```python
from build123d import *

# Parameters (mm, degrees)
EXTRUDE_1_DEPTH = 10
EXTRUDE_2_DEPTH = 2.5
EXTRUDE_3_DEPTH = 2.5


with BuildPart() as part:
    # 草图1 → 凸台-拉伸1 (new body)
    with BuildSketch(Plane.XY):
        Polygon((-6, -2.715432056), (-6, -10.574613101), (-11, -10.574613101), (-11, 19.425386899), (-5, 19.425386899), (5, 19.425386899), (11, 19.425386899), (11, -10.574613101), (6, -10.574613101), (6, -2.715432056), (7, -2.715432056), (7, 14.925386899), (-7, 14.925386899), (-7, -2.715432056), align=None)
    extrude(amount=EXTRUDE_1_DEPTH)

    # 草图2 → 凸台-拉伸2 (add)
    with BuildSketch(Plane(origin=(0, 0, 0), x_dir=(0, 0, -1), z_dir=(1, 0, 0))):
        Polygon((-10, 19.425386899), (-10, 31.425386899), (-14.821209098, 31.425386899), (-14.821209098, 33.063700588), (4.821209098, 33.063700588), (4.821209098, 31.425386899), (0, 31.425386899), (0, 19.425386899), align=None)
    extrude(amount=EXTRUDE_2_DEPTH)

    # 草图2<2> → 凸台-拉伸3 (add)
    with BuildSketch(Plane(origin=(0, 0, 0), x_dir=(0, 0, -1), z_dir=(1, 0, 0))):
        Polygon((-10, 19.425386899), (-10, 31.425386899), (-14.821209098, 31.425386899), (-14.821209098, 33.063700588), (4.821209098, 33.063700588), (4.821209098, 31.425386899), (0, 31.425386899), (0, 19.425386899), align=None)
    extrude(amount=-EXTRUDE_3_DEPTH)


solid = part.part
```
Check sheet for the modelled part. Datum: model origin and axes. Units: mm. A direction names the side the tool comes from. Give positions to 0.01 mm unless a question says otherwise; leave off trailing zeros. Order: outer loops, then holes, each group sorted by start corner. A loop starts at its lowest first (then second) coordinate and runs counter-clockwise, first axis right, second up. Notation, with made-up numbers: M 40,47 L 95,47 A13 cw 95,53 Z; hole C -2,-25.5 d11. An arc over 180 degrees is marked long. Answer in a Markdown table with one row per item. Add a question column.
Q1. Sectioned sample at B-B, the plane z = 6.25. Record the boundary of the cut face in (x, y), and give its area (3 significant figures).
Q2. Release check for a two-part mould opening along Y. For faces 1 (the flat face through (2.5, 26, 5)), 2 (the flat face through (-7, 6, 5)), 3 (the flat face through (7, 6, 5)), 4 (the flat face through (0, 33.064, 5)) record: released by +Y, released by -Y, zero draft, split by the parting line, or undercut.
Q3. Sectioned sample at C-C, the plane y = -7.5. Record the boundary of the cut face in (x, z).
Q4. Gauge pin test, flat ends, axial feed: pin 1 Ø4 at (x, z) = (-8.5, -1.5) entering from +Y; pin 2 Ø7 at (y, z) = (29.5, 8.5) entering from -X; pin 3 Ø3 at (x, z) = (-1.5, 6.5) entering from -Y. Record the tip position at first contact, or that the pin passes through.
Q5. Thickness scan on L1, parallel to X at y = 7, z = 2; L2, parallel to Y at x = -6.5, z = 9.25; L3, parallel to Y at x = -1, z = -3.25. Record the ranges inside material, lowest first.
Q6. Sectioned sample at D-D, the plane x = 7.5. Record the boundary of the cut face in (y, z), and give its area (3 significant figures).
Q7. Sectioned sample at A-A, the plane y = 13. Record the boundary of the cut face in (x, z), and give its area (3 significant figures).
Q8. Access from +Z, -Z, +X, -X, +Y, -Y to the whole of each face (thin tool, end or side, straight path). Record for faces 5 (the flat face through (0, 31.425, -2)), 6 (the flat face through (-7, 19.425, 5)), 7 (the flat face through (-7.2, 5.5, 10)).
Verdict:
| question | item | result |
|---|---|---|
| 1 | outline | M -11,-10.57 L -6,-10.57 L -6,-2.72 L -7,-2.72 L -7,14.93 L 7,14.93 L 7,-2.72 L 6,-2.72 L 6,-10.57 L 11,-10.57 L 11,19.43 L 2.5,19.43 L 2.5,33.06 L -2.5,33.06 L -2.5,19.43 L -11,19.43 Z |
| 1 | area | 387 mm² |
| 2 | face 1 | zero draft |
| 2 | face 2 | undercut |
| 2 | face 3 | undercut |
| 2 | face 4 | released by +Y |
| 3 | outline | M -11,0 L -6,0 L -6,10 L -11,10 Z; M 6,0 L 11,0 L 11,10 L 6,10 Z |
| 4 | pin 1 | y = 19.43 |
| 4 | pin 2 | x = -2.5 |
| 4 | pin 3 | y = 14.93 |
| 5 | L1 | -11 to -7, 7 to 11 |
| 5 | L2 | -10.57 to -2.72, 14.93 to 19.43 |
| 5 | L3 | 31.43 to 33.06 |
| 6 | outline | M -10.57,0 L 19.43,0 L 19.43,10 L -10.57,10 Z |
| 6 | area | 300 mm² |
| 7 | outline | M -11,0 L -7,0 L -7,10 L -11,10 Z; M 7,0 L 11,0 L 11,10 L 7,10 Z |
| 7 | area | 80.0 mm² |
| 8 | face 5 | -Z, +X, -X, -Y |
| 8 | face 6 | +Z, -Z, -X, +Y |
| 8 | face 7 | +Z, +X, -X, -Y |
